from build123d import *

# Parameters (mm, degrees)
BOSS_EXTRUDE1_DEPTH = 127
SKETCH2_W           = 25.4
SKETCH2_H           = 6.35
BOSS_EXTRUDE2_DEPTH = 6.35
LPATTERN1_COUNT     = 2
LPATTERN1_PITCH     = 50.8
SKETCH3_R           = 2.0955
CUT_EXTRUDE1_DEPTH  = 6.35
CUT_EXTRUDE2_DEPTH  = 6.35
BOSS_EXTRUDE4_DEPTH = 6.35
LPATTERN3_COUNT     = 3
LPATTERN3_PITCH     = 50.8
BOSS_EXTRUDE5_DEPTH = 6.35
LPATTERN4_COUNT     = 3
LPATTERN4_PITCH     = 50.8
CUT_EXTRUDE3_DEPTH  = 6.35


with BuildPart() as part:
    # Sketch1 → Boss-Extrude1 (new body)
    with BuildSketch(Plane.XY):
        Polygon((0, 127), (4.490128061, 122.509871939), (-118.019743879, 0), (-122.509871939, 4.490128061), align=None)
    extrude(amount=BOSS_EXTRUDE1_DEPTH)

    # Sketch2 → Boss-Extrude2 (add)
    with BuildSketch(Plane(origin=(-59.009871939, -59.009871939, 0), x_dir=(0, 0, 1), z_dir=(-0.7071067811865474, -0.7071067811865477, 0))):
        with Locations((38.1, 86.627561211)):
            Rectangle(SKETCH2_W, SKETCH2_H)
    boss_extrude2 = extrude(amount=BOSS_EXTRUDE2_DEPTH)

    # LPattern1: Boss-Extrude2 ×2
    with Locations(*[(0, 0, i * LPATTERN1_PITCH) for i in range(1, LPATTERN1_COUNT)]):
        add(boss_extrude2)

    # Sketch3 → Cut-Extrude1 (cut)
    with BuildSketch(Plane(origin=(-59.009871939, 59.009871939, 0), x_dir=(0, 0, -1), z_dir=(0.7071067811865476, -0.7071067811865476, 0))):
        with Locations(Location((-38.1, -86.627561211, 0), (0, 0, 90))):
            Circle(SKETCH3_R)
        with Locations(Location((-88.979711059, -86.627561211, 0), (0, 0, 90))):
            Circle(SKETCH3_R)
    extrude(amount=-CUT_EXTRUDE1_DEPTH, mode=Mode.SUBTRACT)

    # Sketch4 → Cut-Extrude2 (cut)
    with BuildSketch(Plane(origin=(-63.5, 63.5, 0), x_dir=(0, 0, 1), z_dir=(-0.7071067811865476, 0.7071067811865476, 0))):
        Polygon((10.5664, -83.452561211), (14.8336, -83.452561211), (14.8336, -74.689561211), (17.145, -74.689561211), (17.145, -71.514561211), (14.8336, -71.514561211), (14.8336, -68.212561211), (10.5664, -68.212561211), (10.5664, -71.514561211), (8.255, -71.514561211), (8.255, -74.689561211), (10.5664, -74.689561211), align=None)
        Polygon((112.1664, -83.452561211), (116.4336, -83.452561211), (116.4336, -74.689561211), (118.745, -74.689561211), (118.745, -71.514561211), (116.4336, -71.514561211), (116.4336, -68.212561211), (112.1664, -68.212561211), (112.1664, -71.514561211), (109.855, -71.514561211), (109.855, -74.689561211), (112.1664, -74.689561211), align=None)
    extrude(amount=-CUT_EXTRUDE2_DEPTH, mode=Mode.SUBTRACT)

    # Sketch6 → Boss-Extrude4 (add)
    with BuildSketch(Plane(origin=(0, 0, 0), x_dir=(-1, 0, 0), z_dir=(0, 0, -1))):
        Polygon((13.470384182, 104.549359697), (17.960512242, 109.039487758), (35.921024484, 91.078975516), (31.430896424, 86.588847455), align=None)
    boss_extrude4 = extrude(amount=BOSS_EXTRUDE4_DEPTH)

    # LPattern3: Boss-Extrude4 ×3
    with Locations(*[Vector(-0.7071067811865481, -0.7071067811865469, 0) * (i * LPATTERN3_PITCH) for i in range(1, LPATTERN3_COUNT)]):
        add(boss_extrude4)

    # Sketch7 → Boss-Extrude5 (add)
    with BuildSketch(Plane.XY.offset(127)):
        Polygon((-17.960512242, 109.039487758), (-13.470384182, 104.549359697), (-31.430896424, 86.588847455), (-35.921024484, 91.078975516), align=None)
    boss_extrude5 = extrude(amount=BOSS_EXTRUDE5_DEPTH)

    # LPattern4: Boss-Extrude5 ×3
    with Locations(*[Vector(-0.7071067811865475, -0.7071067811865476, 0) * (i * LPATTERN4_PITCH) for i in range(1, LPATTERN4_COUNT)]):
        add(boss_extrude5)

    # Sketch8 → Cut-Extrude3 (cut)
    with BuildSketch(Plane(origin=(-63.5, 63.5, 0), x_dir=(0, 0, 1), z_dir=(-0.7071067811865476, 0.7071067811865476, 0))):
        Polygon((127, -26.631038789), (127, -22.363838789), (118.237, -22.363838789), (118.237, -20.052438789), (115.062, -20.052438789), (115.062, -22.363838789), (111.76, -22.363838789), (111.76, -26.631038789), (115.062, -26.631038789), (115.062, -28.942438789), (118.237, -28.942438789), (118.237, -26.631038789), align=None)
        Polygon((0, 79.236161211), (0, 74.968961211), (8.763, 74.968961211), (8.763, 72.657561211), (11.938, 72.657561211), (11.938, 74.968961211), (15.24, 74.968961211), (15.24, 79.236161211), (11.938, 79.236161211), (11.938, 81.547561211), (8.763, 81.547561211), (8.763, 79.236161211), align=None)
        Polygon((0, -22.363838789), (0, -26.631038789), (8.763, -26.631038789), (8.763, -28.942438789), (11.938, -28.942438789), (11.938, -26.631038789), (15.24, -26.631038789), (15.24, -22.363838789), (11.938, -22.363838789), (11.938, -20.052438789), (8.763, -20.052438789), (8.763, -22.363838789), align=None)
        Polygon((127, 74.968961211), (127, 79.236161211), (118.237, 79.236161211), (118.237, 81.547561211), (115.062, 81.547561211), (115.062, 79.236161211), (111.76, 79.236161211), (111.76, 74.968961211), (115.062, 74.968961211), (115.062, 72.657561211), (118.237, 72.657561211), (118.237, 74.968961211), align=None)
    extrude(amount=-CUT_EXTRUDE3_DEPTH, mode=Mode.SUBTRACT)


solid = part.part
Geometry: final body of the model. Coordinates: model frame, mm. A direction names the side the tool comes from. Round coordinates to 2 decimals unless told otherwise and drop trailing zeros. Loops run counter-clockwise (first coordinate to the right, second up) from the corner with the lowest first, then second, coordinate; pieces in that order, holes last. Notation, with made-up numbers: M 26,28 L 73,28 A8 cw 73,32 Z; hole C 14.5,3.5 d5. An arc over 180 degrees is marked long. Put each result on its own line as item: value. Start each with the question number.
(1) Draft query along Z for faces 1 (the face through (-111, 12, 112.166)), 2 (the face through (-9.91, 112.663, 10.328)), 3 (the face through (-69.628, 52.944, -3.131)), 4 (the face through (-42, 80, 127)). Return one class per face: +Z half, -Z half, draft (parallel to the pull), parting line (faces both ways), or undercut.
(2) Material intervals for line 1 along X through (y, z) = (84, 48.5); line 2 along X through (y, z) = (50, 19); line 3 along Y through (x, z) = (-62, 79.5), sorted ascending. Write a range as [from, to].
(3) Section query D-D (z = 21.5). Return loops of the section in (x, y), then the cut area to 3 significant figures.
(4) Set-up query: faces 5 (the face through (-12, 111, 0)), 6 (the face through (-113, 10, 118.745)), 7 (the face through (-15.75, 106.83, 130.13)), 8 (the face through (-77.1, 45.47, 122.68)), 9 (the face through (-75.47, 47.11, 116.67)). Return all of +Z, -Z, +X, -X, +Y, -Y with unobstructed straight access to the full face (end or side cutting, diameter ignored); none if empty.
(5) Section query B-B (y = 28.5). Return loops of the section in (x, z).
(6) Section query C-C (x = -20.5). Return loops of the section in (y, z).
(7) Section query A-A (z = 48). Return loops of the section in (x, y), then the cut area to 3 significant figures.
(8) Contact query for flat-ended pins moving along their axis: pin 1 Ø5 at (x, z) = (-9.5, 73.5) entering from +Y; pin 2 Ø2.5 at (x, y) = (-120.5, -1.5) entering from +Z; pin 3 Ø6 at (x, y) = (-73.5, 49) entering from -Z; pin 4 Ø24.5 at (x, y) = (-40.5, 75) entering from +Z. Output: stop coordinate, or through.
Findings below:
1. face 1: undercut
1. face 2: undercut
1. face 3: draft
1. face 4: +Z half
2. line 1: x = [-43, -34.02]
2. line 2: x = [-77, -68.02]
2. line 3: y = [56.02, 65]
3. outline: M -122.51,4.49 L -118.02,0 L 4.49,122.51 L 0,127 Z
3. area: 1,100 mm2
4. face 5: -Z, +X, +Y
4. face 6: none
4. face 7: +Z, +X, +Y
4. face 8: +Z
4. face 9: -X, -Y
5. outline: M -98.5,-6.35 L -89.52,-6.35 L -89.52,133.35 L -98.5,133.35 Z
6. outline: M 97.52,-6.35 L 106.5,-6.35 L 106.5,133.35 L 97.52,133.35 Z
7. outline: M -127,0 L -122.51,-4.49 L 4.49,122.51 L 0,127 Z
7. area: 1,140 mm2
8. pin 1: stops at y = 120
8. pin 2: stops at z = 101.6
8. pin 3: stops at z = 0
8. pin 4: stops at z = 133.35
